from build123d import *

# Parameters (mm, degrees)
AUFSATZ_LINEAR_AUSTRAGEN1_DEPTH  = 10
AUFSATZ_LINEAR_START             = 2
AUFSATZ_LINEAR_AUSTRAGEN2_DEPTH  = 2
SKIZZE3_R                        = 2.15
SCHNITT_LINEAR_AUSTRAGEN1_DEPTH  = 63.032572089
SKIZZE5_R                        = 3.7
SKIZZE5_R_2                      = 2.15
SCHNITT_LINEAR_AUSTRAGEN3_DEPTH  = 6
VERRUNDUNG3_START                = -11
VERRUNDUNG3_DEPTH                = 12
VERRUNDUNG3_START_2              = -10.2
VERRUNDUNG3_2_DEPTH              = 10.2
SKIZZE9_W                        = 10
SKIZZE9_H                        = 5
SCHNITT_LINEAR_AUSTRAGEN6_DEPTH  = 62.676900052
SKIZZE10_W                       = 10
SKIZZE10_H                       = 10
AUFSATZ_LINEAR_AUSTRAGEN3_DEPTH  = 5
AUFSATZ_LINEAR_AUSTRAGEN4_DEPTH  = 10
SKIZZE12_R                       = 1.7
SCHNITT_LINEAR_AUSTRAGEN7_DEPTH  = 62.262060037
SCHNITT_LINEAR_AUSTRAGEN8_DEPTH  = 63.032572089
SCHNITT_LINEAR_AUSTRAGEN10_DEPTH = 63.032572089
VERRUNDUNG6_R                    = 5
VERRUNDUNG7_R                    = 12
SCHNITT_LINEAR_AUSTRAGEN11_DEPTH = 6
SKIZZE19_W                       = 48.79312263
SKIZZE19_H                       = 28.151116142
SCHNITT_LINEAR_AUSTRAGEN12_DEPTH = 4
AUFSATZ_LINEAR_AUSTRAGEN6_DEPTH  = 8
VERRUNDUNG8_R                    = 2


with BuildPart() as part:
    # Skizze1 → Aufsatz-Linear austragen1 (new body)
    with BuildSketch(Plane(origin=(0, 0, 0), x_dir=(1, 0, 0), z_dir=(0, 1, 0))):
        with BuildLine():
            Line((-60, 0), (60, 0))
            Line((60, 0), (60, 10.2))
            Line((60, 10.2), (14.486956443, 10.2))
            ThreePointArc((14.486956443, 10.2), (7.840151577, 5.759336515), (0, 4.2))
            ThreePointArc((0, 4.2), (-7.840151577, 5.759336515), (-14.486956443, 10.2))
            Line((-14.486956443, 10.2), (-60, 10.2))
            Line((-60, 10.2), (-60, 0))
        make_face()
    extrude(amount=AUFSATZ_LINEAR_AUSTRAGEN1_DEPTH)

    # Skizze7 → Aufsatz-Linear austragen2 (add)
    with BuildSketch(Plane.XZ.offset(AUFSATZ_LINEAR_START)):
        with BuildLine():
            Line((23, 0), (23, -10.2))
            Line((23, -10.2), (14.486956443, -10.2))
            ThreePointArc((14.486956443, -10.2), (0, -4.2), (-14.486956443, -10.2))
            Line((-14.486956443, -10.2), (-23, -10.2))
            Line((-23, -10.2), (-23, 0))
            Line((-23, 0), (23, 0))
        make_face()
    extrude(amount=-AUFSATZ_LINEAR_AUSTRAGEN2_DEPTH)

    # Skizze3 → Schnitt-Linear austragen1 (cut, through all)
    with BuildSketch(Plane(origin=(0, 10, 0), x_dir=(1, 0, 0), z_dir=(0, 1, 0))):
        with Locations(Location((17.5, 5.2, 0), (0, 0, 270))):
            Circle(SKIZZE3_R)
    extrude(amount=-SCHNITT_LINEAR_AUSTRAGEN1_DEPTH, mode=Mode.SUBTRACT)

    # Skizze5 → Schnitt-Linear austragen3 (cut)
    with BuildSketch(Plane(origin=(0, 10, 0), x_dir=(1, 0, 0), z_dir=(0, 1, 0))):
        with Locations(Location((17.5, 5.2, 0), (0, 0, 270))):
            Circle(SKIZZE5_R)
        with Locations(Location((17.5, 5.2, 0), (0, 0, 270))):
            Circle(SKIZZE5_R_2, mode=Mode.SUBTRACT)
    extrude(amount=-SCHNITT_LINEAR_AUSTRAGEN3_DEPTH, mode=Mode.SUBTRACT)

    # Verrundung3: read off the stored shape, not the designer's step
    # Verrundung3 outline → Verrundung3 (cut)
    with BuildSketch(Plane.XY.offset(VERRUNDUNG3_START)):
        with BuildLine():
            ThreePointArc((23, -1), (22.707106781, -1.707106781), (22, -2))
            Line((22, -2), (23, -2))
            Line((23, -2), (23, -1))
        make_face()
        with BuildLine():
            ThreePointArc((-22, -2), (-22.707106781, -1.707106781), (-23, -1))
            Line((-23, -1), (-23, -2))
            Line((-23, -2), (-22, -2))
        make_face()
    extrude(amount=VERRUNDUNG3_DEPTH, mode=Mode.SUBTRACT)

    # Verrundung3 2 outline → Verrundung3 2 (add)
    with BuildSketch(Plane.XY.offset(VERRUNDUNG3_START_2)):
        with BuildLine():
            Line((-23, 0), (-24, 0))
            ThreePointArc((-24, 0), (-23.292893219, -0.292893219), (-23, -1))
            Line((-23, -1), (-23, 0))
        make_face()
        with BuildLine():
            Line((23, 0), (23, -1))
            ThreePointArc((23, -1), (23.292893219, -0.292893219), (24, 0))
            Line((24, 0), (23, 0))
        make_face()
    extrude(amount=VERRUNDUNG3_2_DEPTH)

    # Skizze9 → Schnitt-Linear austragen6 (cut, through all)
    with BuildSketch(Plane.XY):
        with Locations((-55, 7.5)):
            Rectangle(SKIZZE9_W, SKIZZE9_H)
        with Locations((55, 7.5)):
            Rectangle(SKIZZE9_W, SKIZZE9_H)
    extrude(amount=-SCHNITT_LINEAR_AUSTRAGEN6_DEPTH, mode=Mode.SUBTRACT)

    # Skizze10 → Aufsatz-Linear austragen3 (add)
    with BuildSketch(Plane.XZ):
        with Locations((-55, 5)):
            Rectangle(SKIZZE10_W, SKIZZE10_H)
        with Locations((55, 5)):
            Rectangle(SKIZZE10_W, SKIZZE10_H)
    extrude(amount=-AUFSATZ_LINEAR_AUSTRAGEN3_DEPTH)

    # Skizze11 → Aufsatz-Linear austragen4 (add)
    with BuildSketch(Plane.XY):
        with BuildLine():
            Line((-50, 10), (-50, 0))
            Line((-50, 0), (-24, 0))
            ThreePointArc((-24, 0), (-23.292893219, -0.292893219), (-23, -1))
            ThreePointArc((-23, -1), (-22.707106781, -1.707106781), (-22, -2))
            Line((-22, -2), (22, -2))
            ThreePointArc((22, -2), (22.707106781, -1.707106781), (23, -1))
            ThreePointArc((23, -1), (23.292893219, -0.292893219), (24, 0))
            Line((24, 0), (50, 0))
            Line((50, 0), (50, 10))
            Line((50, 10), (-50, 10))
        make_face()
    extrude(amount=AUFSATZ_LINEAR_AUSTRAGEN4_DEPTH)

    # Skizze12 → Schnitt-Linear austragen7 (cut, through all)
    with BuildSketch(Plane(origin=(0, 5, 0), x_dir=(1, 0, 0), z_dir=(0, 1, 0))):
        with Locations(Location((55, 5.15, 0), (0, 0, 270))):
            Circle(SKIZZE12_R)
        with Locations(Location((55, -4.95, 0), (0, 0, 270))):
            Circle(SKIZZE12_R)
        with Locations(Location((-55, -4.95, 0), (0, 0, 90))):
            Circle(SKIZZE12_R)
        with Locations(Location((-55, 5.15, 0), (0, 0, 90))):
            Circle(SKIZZE12_R)
    extrude(amount=-SCHNITT_LINEAR_AUSTRAGEN7_DEPTH, mode=Mode.SUBTRACT)

    # Skizze14 → Schnitt-Linear austragen8 (cut, through all)
    with BuildSketch(Plane.XZ.offset(2)):
        with BuildLine():
            ThreePointArc((-17.852169734, 6.216943335), (-19.197790162, 0.578814515), (-19.65, -5.2))
            ThreePointArc((-19.65, -5.2), (-17.5, -7.35), (-15.35, -5.2))
            ThreePointArc((-15.35, -5.2), (-14.950132082, -0.090065766), (-13.760263143, 4.895466718))
            ThreePointArc((-13.760263143, 4.895466718), (-15.145478129, 7.602158322), (-17.852169734, 6.216943335))
        make_face()
    extrude(amount=-SCHNITT_LINEAR_AUSTRAGEN8_DEPTH, mode=Mode.SUBTRACT)

    # Skizze15 → Schnitt-Linear austragen10 (cut, through all)
    with BuildSketch(Plane.XZ.offset(2)):
        with BuildLine():
            Line((15.834683057, -10.2), (10.771946853, -14.532947046))
            Line((10.771946853, -14.532947046), (0, -16.110649456))
            Line((0, -16.110649456), (-10.771946853, -14.532947046))
            Line((-10.771946853, -14.532947046), (-15.834683057, -10.2))
            ThreePointArc((-15.834683057, -10.2), (-9.044172408, -1.504818286), (0, 4.813422401))
            ThreePointArc((0, 4.813422401), (9.044172408, -1.504818286), (15.834683057, -10.2))
        make_face()
    extrude(amount=-SCHNITT_LINEAR_AUSTRAGEN10_DEPTH, mode=Mode.SUBTRACT)

    # Verrundung6
    verrundung6_edges = [part.edges().sort_by_distance(p)[0] for p in [
        (15.834683057, 4, -10.2),
        (-15.834683057, 4, -10.2),
    ]]
    fillet(verrundung6_edges, radius=VERRUNDUNG6_R)

    # Verrundung7
    verrundung7_edges = [part.edges().sort_by_distance(p)[0] for p in [
        (0, 4, 4.813422401),
    ]]
    fillet(verrundung7_edges, radius=VERRUNDUNG7_R)

    # Skizze16 → Schnitt-Linear austragen11 (cut)
    with BuildSketch(Plane(origin=(0, 10, 0), x_dir=(1, 0, 0), z_dir=(0, 1, 0))):
        with BuildLine():
            ThreePointArc((-21.15, 5.2), (-20.679531353, -0.812144845), (-19.27957901, -6.677923551))
            ThreePointArc((-19.27957901, -6.677923551), (-14.684497914, -9.029567598), (-12.332853867, -4.434486502))
            ThreePointArc((-12.332853867, -4.434486502), (-13.468390891, 0.323396096), (-13.85, 5.2))
            ThreePointArc((-13.85, 5.2), (-17.5, 8.85), (-21.15, 5.2))
        make_face()
    extrude(amount=-SCHNITT_LINEAR_AUSTRAGEN11_DEPTH, mode=Mode.SUBTRACT)

    # Skizze19 → Schnitt-Linear austragen12 (cut)
    with BuildSketch(Plane.XZ.offset(2)):
        Rectangle(SKIZZE19_W, SKIZZE19_H)
    extrude(amount=-SCHNITT_LINEAR_AUSTRAGEN12_DEPTH, mode=Mode.SUBTRACT)

    # Skizze18 → Aufsatz-Linear austragen6 (add)
    with BuildSketch(Plane.XZ.offset(-2)):
        Polygon((22, -10.2), (22, -24.207768556), (20.316248486, -25.89152007), (18.632496972, -24.207768556), (18.632496972, -10.2), align=None)
    extrude(amount=-AUFSATZ_LINEAR_AUSTRAGEN6_DEPTH)

    # Verrundung8
    verrundung8_edges = [part.edges().sort_by_distance(p)[0] for p in [
        (18.632496972, 6, -10.2),
        (22, 6, -10.2),
    ]]
    fillet(verrundung8_edges, radius=VERRUNDUNG8_R)


solid = part.part
Design review of the part built by this model. Coordinates are the model's own, in mm. A direction names the side the tool comes from. Coordinates: 2 decimals unless noted, no trailing zeros. Order: outer loops, then holes, each group sorted by start corner. A loop starts at its lowest first (then second) coordinate and runs counter-clockwise, first axis right, second up.
Item 1: For faces 1 (the cylindrical face through (-13.46, 7.04, -0.26)), 2 (the flat face through (55, 5, 0)), 3 (the flat face through (-40, 5, -10.2)), 4 (the flat face through (24.397, 1, 0)), list the 3-axis set-ups (+Z, -Z, +X, -X, +Y, -Y) from which the entire face can be reached by the end or side of a thin tool; tool diameter is ignored.
Item 2: Take a section at B-B, the plane y = 8. Count the separate pieces of the cut face and the enclosed holes in it, then the cut area to 3 significant figures.
Item 3: For line 1 (X direction, y = 1.1, z = 4.95); line 2 (X direction, y = 4.25, z = -2.5); line 3 (Y direction, x = 19, z = -1.5), list the stretches that pass through material, from the lowest coordinate up.
Item 4: Take a section at A-A, the plane x = -55. Write out the cut boundary in (y, z), then the cut area to 3 significant figures.
Item 5: Take a section at C-C, the plane x = -42.5. Write out the cut boundary in (y, z), then the cut area to 3 significant figures.
Item 6: The part is to be moulded in two halves that separate along X. For faces 5 (the flat face through (-55, 5, 0)), 6 (the flat face through (-24.397, 1, 0)), 7 (the flat face through (60, 2, 0)), say which applies: pulls with the +X half, pulls with the -X half, needs draft (parallel to the pull), parting line crosses it, or undercut.
Item 7: For pin 1 Ø2.5 at (y, z) = (5.5, -21) entering from +X; pin 2 Ø2.5 at (y, z) = (7, -5) entering from -X; pin 3 Ø1 at (y, z) = (1, -21.5) entering from -X; pin 4 Ø4 at (y, z) = (5, -17) entering from -X, all flat-tipped, find the tip position at first contact; note any pin that passes through.
The answers:
1. face 1: +Y
1. face 2: +Z, -Z, +X, +Y
1. face 3: -Z, -X, +Y, -Y
1. face 4: +Z, -Z, -Y
2. separate pieces: 1
2. enclosed holes: 2
2. area: 1,630 mm2
3. line 1: x = -60 to -56.7, -53.3 to -24.4, 24.4 to 53.3, 56.7 to 60
3. line 2: x = -60 to -21.06, -13.73 to -10.05, 10.05 to 14.97, 20.03 to 60
3. line 3: y = 2 to 10
4. outline: (0, -10.2) - (5, -10.2) - (5, -6.85) - (0, -6.85) - close; (0, -3.45) - (5, -3.45) - (5, 3.25) - (0, 3.25) - close; (0, 6.65) - (5, 6.65) - (5, 10) - (0, 10) - close
4. area: 67.0 mm2
5. outline: (0, -10.2) - (10, -10.2) - (10, 10) - (0, 10) - close
5. area: 202 mm2
6. face 5: needs draft
6. face 6: undercut
6. face 7: pulls with the +X half
7. pin 1: stops at x = 22
7. pin 2: stops at x = -50
7. pin 3: passes through
7. pin 4: stops at x = 18.63
